Input: part model. Units: mm. Frame: model coordinates. A direction names the side the tool comes from. Coordinates: 2 decimals unless noted, no trailing zeros. Loops run counter-clockwise (first coordinate to the right, second up) from the corner with the lowest first, then second, coordinate; pieces in that order, holes last. Notation, with made-up numbers: (-4, -19) -> (24, -19) arc R15 cw to (24, 7) -> close; hole circle Ø8 at (57.25, 56). An arc over 180 degrees is marked (long way). Answer as a JSON object with one key per item and string values.
from build123d import *

# Parameters (mm, degrees)
F0_W     = 63.5
F0_H     = 79.375
F0_W_2   = 60.325
F0_H_2   = 76.2
F1_DEPTH = 30.1625
F2_W     = 60.325
F2_H     = 1.5875
F3_DEPTH = 76.2
F4_W     = 12.7
F4_H     = 15.875
F5_DEPTH = 1.5875
F6_W     = 12.7
F6_H     = 15.875
F7_DEPTH = 1.5875


with BuildPart() as f1:
    # F0 (on Top) → F1 (new body)
    with BuildSketch(Plane.XY):
        with Locations((31.75, 39.6875)):
            Rectangle(F0_W, F0_H)
        with Locations((31.75, 39.6875)):
            Rectangle(F0_W_2, F0_H_2, mode=Mode.SUBTRACT)
    extrude(amount=F1_DEPTH)

    # F2 (on face) → F3 (join)
    with BuildSketch(Plane.XZ.offset(-77.7875)):
        with Locations((31.75, 29.36875)):
            Rectangle(F2_W, F2_H)
    extrude(amount=F3_DEPTH)

    # F4 (on face) → F5 (cut)
    with BuildSketch(Plane.XY.offset(30.1625)):
        with Locations((33.3375, 63.5)):
            Rectangle(F4_W, F4_H)
    extrude(amount=-F5_DEPTH, mode=Mode.SUBTRACT)

    # F6 (on face) → F7 (cut)
    with BuildSketch(Plane.XZ):
        with Locations((17.4625, 7.9375)):
            Rectangle(F6_W, F6_H)
    extrude(amount=-F7_DEPTH, mode=Mode.SUBTRACT)


solid = f1.part
1. Section query C-C (y = 49.5). Return loops of the section in (x, z) (1 decimal), plus the area to 3 significant figures.
Reply:
{"outline": "(0, 0) -> (1.6, 0) -> (1.6, 28.6) -> (61.9, 28.6) -> (61.9, 0) -> (63.5, 0) -> (63.5, 30.2) -> (0, 30.2) -> close", "area": "192 mm2"}
2. Section query D-D (z = 14.5). Return loops of the section in (x, y) (1 decimal).
Reply:
{"outline": "(0, 0) -> (11.1, 0) -> (11.1, 1.6) -> (1.6, 1.6) -> (1.6, 77.8) -> (61.9, 77.8) -> (61.9, 1.6) -> (23.8, 1.6) -> (23.8, 0) -> (63.5, 0) -> (63.5, 79.4) -> (0, 79.4) -> close"}
3. Section query A-A (y = 66). Return loops of the section in (x, z) (1 decimal), plus the area to 3 significant figures.
Reply:
{"outline": "(0, 0) -> (1.6, 0) -> (1.6, 28.6) -> (27, 28.6) -> (27, 30.2) -> (0, 30.2) -> close; (39.7, 28.6) -> (61.9, 28.6) -> (61.9, 0) -> (63.5, 0) -> (63.5, 30.2) -> (39.7, 30.2) -> close", "area": "171 mm2"}
4. Section query B-B (z = 26). Return loops of the section in (x, y) (1 decimal), plus the area to 3 significant figures.
Reply:
{"outline": "(0, 0) -> (63.5, 0) -> (63.5, 79.4) -> (0, 79.4) -> close; hole (1.6, 1.6) -> (61.9, 1.6) -> (61.9, 77.8) -> (1.6, 77.8) -> close", "area": "444 mm2"}
5. Line query: line 1 along Y through (x, z) = (60, 17) (1 decimal); line 2 along X through (y, z) = (32.5, 12.5); line 3 along Z through (x, y) = (58, 69) (1 decimal). Output: solid intervals per line, ascending.
Reply:
{"line 1": "y = 0 to 1.6, 77.8 to 79.4", "line 2": "x = 0 to 1.59, 61.91 to 63.5", "line 3": "z = 28.6 to 30.2"}
6. Access query for faces 4 (the face through (32, 78, 0)), 5 (the face through (31, 77.788, 14)). Directions: +Z, -Z, +X, -X, +Y, -Y. A direction counts if a zero-diameter tool reaches every point of the face in a straight line with its end or side. Return the directions, or none.
Reply:
{"face 4": "-Z, +X, -X, +Y, -Y", "face 5": "-Z"}
7. Pin query (flat end, axial travel): P1, Ø8, axis at x = 13.5, y = 42.5, coming from the -Z side (3 decimals); P2, Ø1.3, axis at x = 19, y = 1, coming from the -Z side (3 decimals). Return the tip coordinate at first contact, or that it passes through.
Reply:
{"P1": "stops at z = 28.575", "P2": "stops at z = 15.875"}
8. Mould query, pull axis Y, two halves, no side actions, for faces 1 (the face through (31, 40, 30.162)), 2 (the face through (31, 79.375, 15)), 3 (the face through (61.912, 39, 14)). Classes: pulls with the +Y half, pulls with the -Y half, needs draft (parallel to the pull), parting line crosses it, or undercut.
Reply:
{"face 1": "needs draft", "face 2": "pulls with the +Y half", "face 3": "undercut"}
